```python
from build123d import *

# Parameters (mm, degrees)
BOSS_EXTRUDE1_DEPTH      = 1.5
BOSS_EXTRUDE1_DEPTH_BACK = 1.5
SKETCH2_R                = 8
SKETCH3_W                = 16
SKETCH3_H                = 30
BOSS_EXTRUDE2_DEPTH      = 1.5
CUT_EXTRUDE1_REACH       = 33.193
SKETCH4_R                = 1.65
CUT_EXTRUDE2_REACH       = 33.193
SKETCH5_R                = 3.5
FILLET1_R                = 1
FILLET2_R                = 3


with BuildPart() as part:
    # Sketch2 → Boss-Extrude1 (new, two sides: drawn at the far end of the back side and taken through both)
    with BuildSketch(Plane(origin=(0, 0, 0), x_dir=(1, 0, 0), z_dir=(0, 1, 0)).offset(-BOSS_EXTRUDE1_DEPTH_BACK)):
        with Locations(Location((0, 0, 0), (0, 0, 270))):
            Circle(SKETCH2_R)
    extrude(amount=BOSS_EXTRUDE1_DEPTH + BOSS_EXTRUDE1_DEPTH_BACK)

    # Sketch3 → Boss-Extrude2 (add, symmetric)
    with BuildSketch(Plane(origin=(0, 0, 0), x_dir=(1, 0, 0), z_dir=(0, 1, 0))):
        with Locations((0, -15)):
            Rectangle(SKETCH3_W, SKETCH3_H)
    extrude(amount=BOSS_EXTRUDE2_DEPTH, both=True)

    # Sketch4 → Cut-Extrude1 (cut, up to next)
    with BuildSketch(Plane(origin=(0, 1.5, 0), x_dir=(1, 0, 0), z_dir=(0, 1, 0)), mode=Mode.PRIVATE) as cut_extrude1_sk1:
        with Locations(Location((2.5, -25.5, 0), (0, 0, 270))):
            Circle(SKETCH4_R)
    cut_extrude1_tool1 = extrude(cut_extrude1_sk1.sketch, amount=-CUT_EXTRUDE1_REACH, mode=Mode.PRIVATE) & part.part
    # Sketch4 → Cut-Extrude1 (cut, up to next)
    with BuildSketch(Plane(origin=(0, 1.5, 0), x_dir=(1, 0, 0), z_dir=(0, 1, 0)), mode=Mode.PRIVATE) as cut_extrude1_sk2:
        with Locations(Location((-2.5, -25.5, 0), (0, 0, 270))):
            Circle(SKETCH4_R)
    cut_extrude1_tool2 = extrude(cut_extrude1_sk2.sketch, amount=-CUT_EXTRUDE1_REACH, mode=Mode.PRIVATE) & part.part
    add(cut_extrude1_tool1.solids().sort_by_distance((2.5, 1.5, 25.5))[0], mode=Mode.SUBTRACT)
    add(cut_extrude1_tool2.solids().sort_by_distance((-2.5, 1.5, 25.5))[0], mode=Mode.SUBTRACT)

    # Sketch5 → Cut-Extrude2 (cut, up to next)
    with BuildSketch(Plane.XZ.offset(1.5), mode=Mode.PRIVATE) as cut_extrude2_sk1:
        with Locations(Location((0, 0, 0), (0, 0, 270))):
            Circle(SKETCH5_R)
    cut_extrude2_tool1 = extrude(cut_extrude2_sk1.sketch, amount=-CUT_EXTRUDE2_REACH, mode=Mode.PRIVATE) & part.part
    add(cut_extrude2_tool1.solids().sort_by_distance((0, -1.5, 0))[0], mode=Mode.SUBTRACT)

    # Fillet1
    fillet1_edges = [part.edges().sort_by_distance(p)[0] for p in [
        (0, 1.5, 3.5),
        (0, -1.5, 3.5),
    ]]
    fillet(fillet1_edges, radius=FILLET1_R)

    # Fillet2
    fillet2_edges = [part.edges().sort_by_distance(p)[0] for p in [
        (-8, 0, 30),
        (8, 0, 30),
    ]]
    fillet(fillet2_edges, radius=FILLET2_R)


solid = part.part
```
Read the model definition and answer for the solid it produces. Units are mm, in the model's axes. Give positions to 0.01 mm unless a question says otherwise; leave off trailing zeros. Write each loop counter-clockwise with the first axis right and the second up, starting at its lowest first coordinate (ties: lowest second). Pieces come first, ordered by that corner, then holes. Notation, with made-up numbers: (2.25, 11.5) -> (32.25, 11.5) arc R12 ccw to (32.25, 30.5) -> close; hole circle Ø4 at (23, -39.75). An arc over 180 degrees is marked (long way). Answer in a Markdown table with one row per item.
1) Section B-B on x = 0 is taken. Give the vertices of the cut face in (y, z), plus the area to 3 significant figures.
Results list:
| item | result |
|---|---|
| outline | (-1.5, -8) -> (1.5, -8) -> (1.5, -4.5) arc R1 ccw to (0.5, -3.5) -> (-0.5, -3.5) arc R1 ccw to (-1.5, -4.5) -> close; (-1.5, 4.5) arc R1 ccw to (-0.5, 3.5) -> (0.5, 3.5) arc R1 ccw to (1.5, 4.5) -> (1.5, 30) -> (-1.5, 30) -> close |
| area | 92.1 mm^2 |
2) Section A-A on y = 0.15 is taken. Give the vertices of the cut face in (x, z).
Results list:
| item | result |
|---|---|
| outline | (-8, 0) arc R8 ccw to (8, 0) -> (8, 27) arc R3 ccw to (5, 30) -> (-5, 30) arc R3 ccw to (-8, 27) -> close; hole circle Ø3.3 at (-2.5, 25.5); hole circle Ø7 at (0, 0); hole circle Ø3.3 at (2.5, 25.5) |
3) Straight lines are drawn through the part: line 1 (X direction, y = -0.45, z = 25.5); line 2 (X direction, y = -0.2, z = 0); line 3 (X direction, y = 0.1, z = 24.5). For each, find the intervals that lie inside material, in ascending order. Write a range as [from, to].
Results list:
| item | result |
|---|---|
| line 1 | [-8, -4.15], [-0.85, 0.85], [4.15, 8] |
| line 2 | [-8, -3.5], [3.5, 8] |
| line 3 | [-8, -3.81], [-1.19, 1.19], [3.81, 8] |
4) Determine the mould class of faces 1 (the cylindrical face through (0, 0, -8)), 2 (the cylindrical face through (-2.43, 0.02, 23.85)), 3 (the flat face through (0, 1.5, 15)) for opening direction Z: released by +Z, released by -Z, zero draft, split by the parting line, or undercut.
Results list:
| item | result |
|---|---|
| face 1 | released by -Z |
| face 2 | undercut |
| face 3 | zero draft |
5) Section C-C on x = -2.5 is taken. Count the separate pieces of the cut face and the enclosed holes in it, plus the area to 3 significant figures.
Results list:
| item | result |
|---|---|
| separate pieces | 3 |
| enclosed holes | 0 |
| area | 87.0 mm^2 |
6) Section D-D on x = -6.25 is taken. Give the vertices of the cut face in (y, z), plus the area to 3 significant figures.
Results list:
| item | result |
|---|---|
| outline | (-1.5, -4.99) -> (1.5, -4.99) -> (1.5, 29.73) -> (-1.5, 29.73) -> close |
| area | 104 mm^2 |
7) This flat-tipped pin is pushed along its axis until it touches: pin 1 Ø2.5 at (x, z) = (2.5, 25.5) entering from +Y. Where does it stop, or does it pass through?
Results list:
| item | result |
|---|---|
| pin 1 | through |
